Source: CAD feature listing. Evaluate the final solid. Frame: model axes, mm. Round coordinates to 2 decimals unless told otherwise and drop trailing zeros. Order: outer loops, then holes, each group sorted by start corner. A loop starts at its lowest first (then second) coordinate and runs counter-clockwise, first axis right, second up. Notation, with made-up numbers: (20.25, 5) - (46.25, 5) arc R17 ccw to (46.25, 29) - close; hole circle Ø2 at (86, 3). An arc over 180 degrees is marked (long way). Use one line per item in the form item = value. Start each with the question number.
Q1. Pin query (flat end, axial travel): pin 1 Ø4.5 at (y, z) = (271.46, 26.95) entering from -X. Return the tip coordinate at first contact, or that it passes through.
Q2. Cut plane A-A, the plane y = 203.2. Return the cut outline in (x, z), and give its area (3 significant figures).
Q3. Ray query, line 1 (Y direction, x = 0.25, z = 33); line 2 (Y direction, x = 0.45, z = 39.5); line 3 (Y direction, x = 0.25, z = 28). Return the intervals inside material, ascending. Write a range as [from, to].
Q4. Draft query along Y for faces 1 (the flat face through (0, 135, 18)), 2 (the cylindrical face through (0.41, 2.46, 12.75)), 3 (the cylindrical face through (0.41, 3.65, 29.09)). Return one class per face: released by +Y, released by -Y, zero draft, split by the parting line, or undercut.
from build123d import *

# Parameters (mm, degrees)
F1_DEPTH = 0.8001
F2_D     = 4.826
F3_D     = 3.81


with BuildPart() as f1:
    # F0 (on Right) → F1 (new body)
    with BuildSketch(Plane.YZ):
        Polygon((274.6375, -12.7), (274.6375, 0), (274.6375, 48.3108), (0, 48.3108), (0, 0), (0, -12.7), align=None)
    extrude(amount=F1_DEPTH)

    # F2 (through all)
    with Locations(Plane(origin=(0, 0, 0), x_dir=(0, 1, 0), z_dir=(-1, 0, 0))):
        with Locations((4.7625, -40.4241), (4.7625, -26.9494), (4.7625, -13.4747), (203.2, -33.1423059973)):
            Hole(F2_D / 2)

    # F3 (through all)
    with Locations(Plane(origin=(0, 0, 0), x_dir=(0, 1, 0), z_dir=(-1, 0, 0))):
        with Locations((271.4625, -40.4241), (271.4625, -26.9494), (271.4625, -13.4747)):
            Hole(F3_D / 2)


solid = f1.part
Completed:
q1.pin_1 = 0
q2.outline = (0, -12.7) - (0.8, -12.7) - (0.8, 30.73) - (0, 30.73) - close; (0, 35.56) - (0.8, 35.56) - (0.8, 48.31) - (0, 48.31) - close
q2.area = 45.0 mm2
q3.line_1 = [0, 200.79], [205.61, 274.64]
q3.line_2 = [0, 2.53], [6.99, 269.8], [273.13, 274.64]
q3.line_3 = [0, 2.59], [6.93, 269.87], [273.05, 274.64]
q4.face_1 = zero draft
q4.face_2 = undercut
q4.face_3 = undercut
